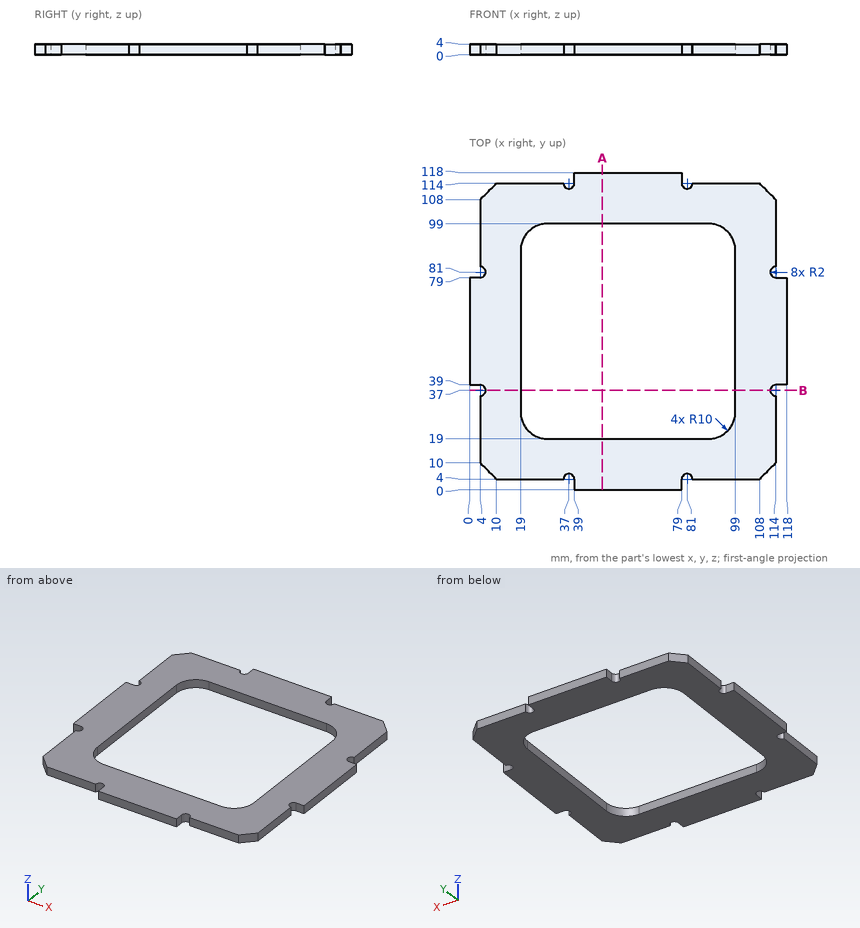
Could you check a few things on this drawing? It's one solid part, dimensions in mm from its lowest x, y, z. Coordinates: 2 decimals unless noted, no trailing zeros. Write each loop counter-clockwise with the first axis right and the second up, starting at its lowest first coordinate (ties: lowest second). Pieces come first, ordered by that corner, then holes. Notation, with made-up numbers: (-16.5, -19.75) - (22.5, -19.75) arc R23 cw to (22.5, -11.75) - close; hole circle Ø4 at (85.5, 5). An arc over 180 degrees is marked (long way). Put each result on its own line as item: value. Start each with the question number.
Q1. I'm going to push flat-ended pins straight in: P1, Ø1.2, axis at x = 25.5, z = 2.5, coming from the +Y side; P2, Ø1.2, axis at y = 3, z = 2.5, coming from the -X side; P3, Ø1.2, axis at x = 116, z = 3, coming from the +Y side; P4, Ø2, axis at x = 81, y = 17, coming from the -Z side. Where does each tip first touch, or does it pass through?
Q2. I want a section at B-B on y = 37. Write out the boundary of the cut face in (x, z).
Q3. I want a section at A-A on x = 49.5. Write out the boundary of the cut face in (y, z).
Q4. Please list where these lines run through material, in increasing order: L1, parallel to X at y = 55, z = 1.75; L2, parallel to Y at x = 30.5, z = 2.2.
Checks:
1. P1: y = 114
1. P2: x = 39
1. P3: y = 79
1. P4: z = 0
2. outline: (6, 0) - (19, 0) - (19, 4) - (6, 4) - close; (99, 0) - (112, 0) - (112, 4) - (99, 4) - close
3. outline: (0, 0) - (19, 0) - (19, 4) - (0, 4) - close; (99, 0) - (118, 0) - (118, 4) - (99, 4) - close
4. L1: 0 to 19, 99 to 118
4. L2: 4 to 19, 99 to 114
